Input: part model. Units: mm. Frame: model coordinates. Face numbers are marked on the shaded views. Round coordinates to 2 decimals unless told otherwise and drop trailing zeros. Loops run counter-clockwise (first coordinate to the right, second up) from the corner with the lowest first, then second, coordinate; pieces in that order, holes last. Notation, with made-up numbers: (-3, 74) -> (22, 74) arc R33 ccw to (22, 109) -> close; hole circle Ø8 at (20, 79). An arc over 180 degrees is marked (long way). Answer as a JSON object with one key per item and string values. Group by question number.
Item 1: Section query A-A on y = 4. Return loops of the section in (x, z) (3 decimals), and give its area (3 significant figures).
Item 2: Draft query along Z for the marked faces 1, 2 and 3. Return one class per face: released by +Z, released by -Z, zero draft, split by the parting line, or undercut.
Item 3: Section query C-C on z = -0.1. Return loops of the section in (x, y) (3 decimals).
Item 4: Material intervals for line 1 (Z direction, x = -0.2, y = -2.75); line 2 (Y direction, x = 0.05, z = -0.95); line 3 (Y direction, x = -0.05, z = -1.25), sorted ascending. Write a range as [from, to].
Item 5: Section query B-B on x = 0.2. Return loops of the section in (y, z) (3 decimals), and give its area (3 significant figures).
Item 6: Section query D-D on y = -3. Return loops of the section in (x, z) (3 decimals), and give its area (3 significant figures).
from build123d import *

# Parameters (mm, degrees)
BOSS_EXTRUDE1_DEPTH      = 0.315
BOSS_EXTRUDE1_DEPTH_BACK = 0.315


with BuildPart() as part:
    # Sketch2 → Boss-Extrude1 (new, two sides: drawn at the far end of the back side and taken through both)
    with BuildSketch(Plane(origin=(0, 0, 0), x_dir=(0, 0, -1), z_dir=(1, 0, 0)).offset(-BOSS_EXTRUDE1_DEPTH_BACK)):
        with BuildLine():
            Line((1.5, 0), (0.595, 0))
            Line((0.595, 0), (0, -5))
            Line((0, -5), (-0.595, 0))
            Line((-0.595, 0), (-1.5, 0))
            Line((-1.5, 0), (-1.5, 4.8))
            ThreePointArc((-1.5, 4.8), (0, 6.3), (1.5, 4.8))
            Line((1.5, 4.8), (1.5, 0))
        make_face()
        with BuildLine():
            Line((-0.8, 3.545), (-0.8, 4.435))
            ThreePointArc((-0.8, 4.435), (0, 5.235), (0.8, 4.435))
            Line((0.8, 4.435), (0.8, 3.545))
            ThreePointArc((0.8, 3.545), (0, 2.745), (-0.8, 3.545))
        make_face(mode=Mode.SUBTRACT)
    extrude(amount=BOSS_EXTRUDE1_DEPTH + BOSS_EXTRUDE1_DEPTH_BACK)


solid = part.part
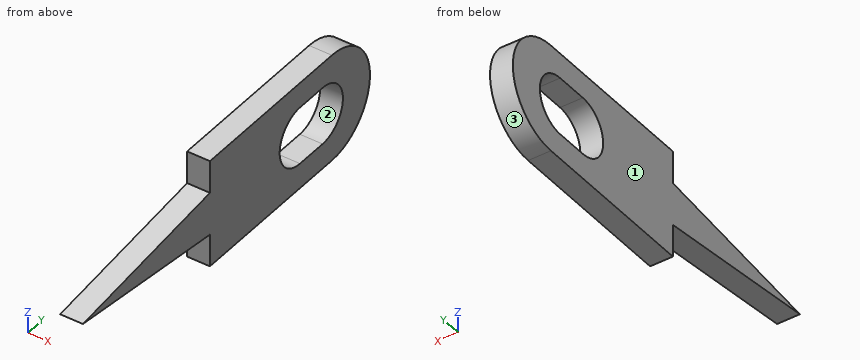
Solved:
{
 "1": {"outline": "(-0.315, -1.5) -> (0.315, -1.5) -> (0.315, -0.8) -> (-0.315, -0.8) -> close; (-0.315, 0.8) -> (0.315, 0.8) -> (0.315, 1.5) -> (-0.315, 1.5) -> close", "area": "0.882 mm²"},
 "2": {"face 1": "zero draft", "face 2": "undercut", "face 3": "split by the parting line"},
 "3": {"outline": "(-0.315, -4.16) -> (0.315, -4.16) -> (0.315, 2.751) -> (-0.315, 2.751) -> close; (-0.315, 5.229) -> (0.315, 5.229) -> (0.315, 6.297) -> (-0.315, 6.297) -> close"},
 "4": {"line 1": "[-0.27, 0.27]", "line 2": "[0, 5.96]", "line 3": "[0, 5.63]"},
 "5": {"outline": "(-5, 0) -> (0, -0.595) -> (0, -1.5) -> (4.8, -1.5) arc R1.5 ccw to (4.8, 1.5) -> (0, 1.5) -> (0, 0.595) -> close; hole (3.545, -0.8) -> (4.435, -0.8) arc R0.8 ccw to (4.435, 0.8) -> (3.545, 0.8) arc R0.8 ccw to start", "area": "17.5 mm²"},
 "6": {"outline": "(-0.315, -0.238) -> (0.315, -0.238) -> (0.315, 0.238) -> (-0.315, 0.238) -> close", "area": "0.300 mm²"}
}
